Can you work these out from the model? Positions are in its coordinate system, mm. Face numbers are marked on the shaded views. Give positions to 0.01 mm unless a question says otherwise; leave off trailing zeros. Loops run counter-clockwise (first coordinate to the right, second up) from the corner with the lowest first, then second, coordinate; pieces in that order, holes last. Notation, with made-up numbers: (-15.5, -40) - (17.5, -40) arc R12 ccw to (17.5, -18) - close; hole circle Ø6 at (0.5, -28). An arc over 180 degrees is marked (long way). Write item = value, one per line.
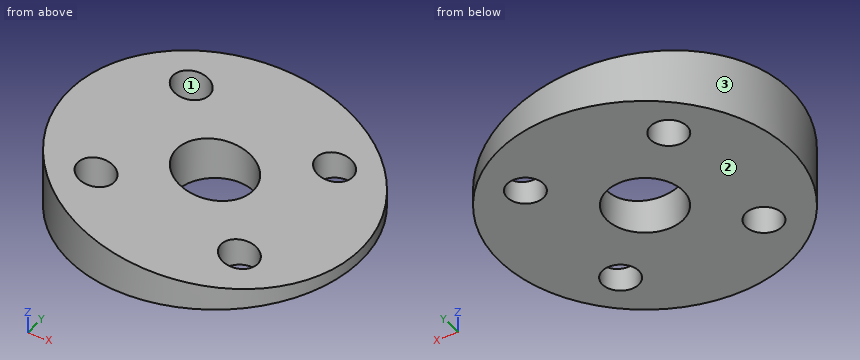
from build123d import *

# Parameters (mm, degrees)
SKETCH1_W           = 41.85
SKETCH1_H           = 10
SKETCH1_W_2         = 10
SKETCH1_H_2         = 29
BOSS_EXTRUDE1_DEPTH = 48
SKETCH4_R           = 2
SKETCH4_R_2         = 4.2
CUT_EXTRUDE2_DEPTH  = 48
SKETCH7_W           = 100.326592526
SKETCH7_H           = 57.143742852
CUT_EXTRUDE5_DEPTH  = 14.7
CUT_EXTRUDE6_DEPTH  = 54.7
BOSS_EXTRUDE5_DEPTH = 13.7
SKETCH19_W          = 55.248240751
SKETCH19_H          = 86.451998217
SKETCH19_R          = 16
CUT_EXTRUDE10_DEPTH = 13.7


with BuildPart() as part:
    # Sketch1 → Boss-Extrude1 (new body)
    with BuildSketch(Plane(origin=(0, 0, 0), x_dir=(1, 0, 0), z_dir=(0, 1, 0))):
        with Locations((-10.925, 5)):
            Rectangle(SKETCH1_W, SKETCH1_H)
        with Locations((5, -14.5)):
            Rectangle(SKETCH1_W_2, SKETCH1_H_2)
    extrude(amount=BOSS_EXTRUDE1_DEPTH)

    # Sketch4 → Cut-Extrude2 (cut)
    with BuildSketch(Plane.XY):
        with Locations((-5.589559388, 40.980827232)):
            Circle(SKETCH4_R)
        with Locations((-5.629681083, 24.979051073)):
            Circle(SKETCH4_R)
        with Locations((-21.591335547, 41.020948927)):
            Circle(SKETCH4_R)
        with Locations((-21.631457243, 25.019172768)):
            Circle(SKETCH4_R)
        with Locations((-13.629681083, 32.979051073)):
            Circle(SKETCH4_R_2)
    extrude(amount=-CUT_EXTRUDE2_DEPTH, mode=Mode.SUBTRACT)

    # Sketch7 → Cut-Extrude5 (cut)
    with BuildSketch(Plane.XZ):
        with Locations((-16.144605738, 7.803574406)):
            Rectangle(SKETCH7_W, SKETCH7_H)
    extrude(amount=-CUT_EXTRUDE5_DEPTH, mode=Mode.SUBTRACT)

    # Sketch8 → Cut-Extrude6 (cut)
    with BuildSketch(Plane.XZ.offset(-14.7)):
        Polygon((-31.85, -2.620715857), (10, -10), (10, 29), (0, 29), (0, 0), (-31.85, 0), align=None)
    extrude(amount=-CUT_EXTRUDE6_DEPTH, mode=Mode.SUBTRACT)

    # Sketch18 → Boss-Extrude5 (add)
    with BuildSketch(Plane(origin=(0, 48, 0), x_dir=(1, 0, 0), z_dir=(0, 1, 0))):
        Polygon((-31.85, 2.620715857), (-31.85, 10), (10, 10), align=None)
    extrude(amount=BOSS_EXTRUDE5_DEPTH)

    # Sketch19 → Cut-Extrude10 (cut)
    with BuildSketch(Plane(origin=(0, 0, -10), x_dir=(-1, 0, 0), z_dir=(0, 0, -1))):
        with Locations((12.788642717, 43.225999109)):
            Rectangle(SKETCH19_W, SKETCH19_H)
        with Locations((13.629681083, 32.979051073)):
            Circle(SKETCH19_R, mode=Mode.SUBTRACT)
    extrude(amount=-CUT_EXTRUDE10_DEPTH, mode=Mode.SUBTRACT)


solid = part.part
Q1. Imagine slicing it at C-C, the plane x = -16. Write out the boundary of the cut face in (y, z), then the cut area to 3 significant figures.
Output:
outline = (17.16, -10) - (29.51, -10) - (29.51, -5.42) - (17.16, -5.42) - close; (36.45, -10) - (48.8, -10) - (48.8, -5.42) - (36.45, -5.42) - close
area = 113 mm2
Q2. Imagine slicing it at D-D, the plane z = -8.25. Write out the boundary of the cut face in (x, y).
Output:
outline = (0.08, 24.72) - (0.08, 41.24) arc R16 ccw (long way) to start; hole circle Ø4 at (-21.63, 25.02); hole circle Ø4 at (-21.59, 41.02); hole circle Ø8.4 at (-13.63, 32.98); hole circle Ø4 at (-5.63, 24.98); hole circle Ø4 at (-5.59, 40.98)
Q3. I need wall thicknesses on L1, parallel to Y at x = -6, z = -9.5; L2, parallel to Y at x = -13.5, z = -6; L3, parallel to X at y = 33, z = -5.5. Which ranges of each line are inside material? Lowest first, please.
Output:
L1 = 18.92 to 23.01, 26.94 to 39.02, 42.94 to 47.04
L2 = 16.98 to 28.78, 37.18 to 48.98
L3 = -29.63 to -17.83
Q4. For pin 1 (2 mm diameter, centred on x = -15, z = -7, fed in from +Y); pin 2 (1 mm diameter, centred on y = 41, z = -4, fed in from -X); pin 3 (6.5 mm diameter, centred on x = -21.63, y = 25.02, fed in from +Z); pin 4 (7.5 mm diameter, centred on x = -13.63, y = 32.98, fed in from -Z), each with a flat end and sliding along its axis, tell me the tip position at first contact or that it passes through.
Output:
pin_1 = 48.97
pin_2 = -27.75
pin_3 = -3.85
pin_4 = through
Q5. Imagine slicing it at A-A, the plane x = -20.5. Write out the boundary of the cut face in (y, z).
Output:
outline = (18.53, -10) - (23.37, -10) - (23.37, -4.62) - (18.53, -4.62) - close; (26.67, -10) - (39.34, -10) - (39.34, -4.62) - (26.67, -4.62) - close; (42.7, -10) - (47.43, -10) - (47.43, -4.62) - (42.7, -4.62) - close
Q6. Imagine slicing it at B-B, the plane y = 34.5. Write out the boundary of the cut face in (x, z) (3 decimals), then the cut area to 3 significant figures.
Output:
outline = (-29.557, -10) - (-17.545, -10) - (-17.545, -5.143) - (-29.557, -3.025) - close; (-9.715, -10) - (2.298, -10) - (2.298, -8.642) - (-9.715, -6.524) - close
area = 100 mm2
Q7. We'd pull the mould along Y, two halves only. Please class the marked faces 1, 2 and 3: released by +Y, released by -Y, zero draft, split by the parting line, or undercut.
Output:
face_1 = undercut
face_2 = zero draft
face_3 = split by the parting line
